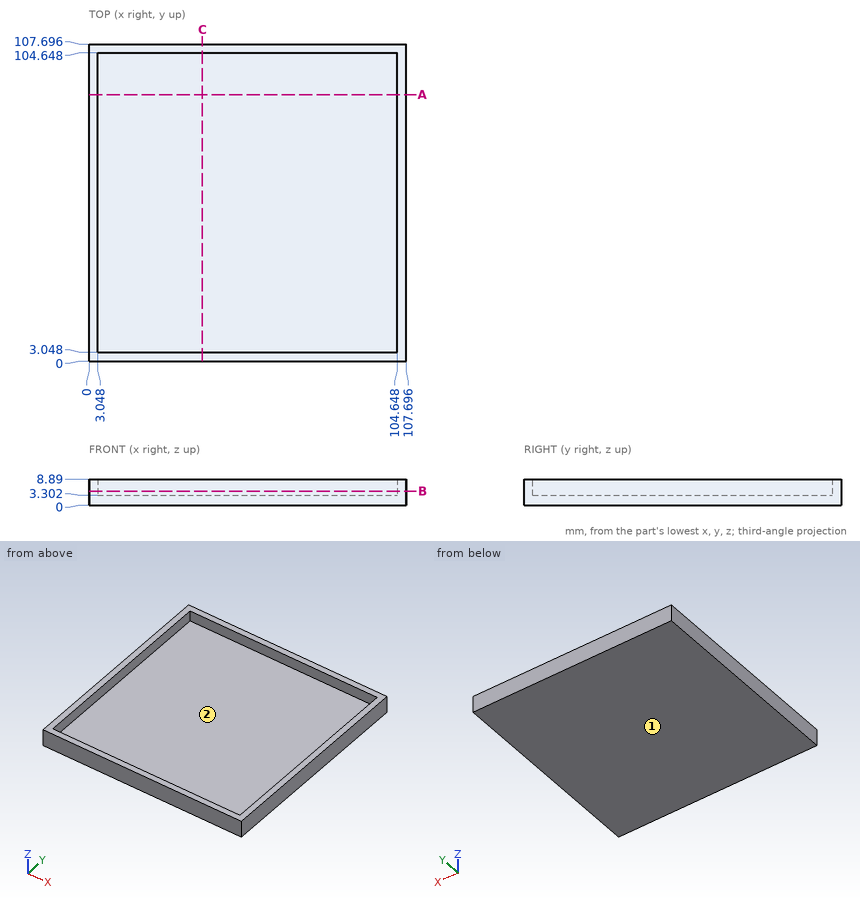
Job drawing, mm, ordinate dimensions from the low corner. One solid piece. Round coordinates to 2 decimals unless told otherwise and drop trailing zeros. Loops run counter-clockwise (first coordinate to the right, second up) from the corner with the lowest first, then second, coordinate; pieces in that order, holes last. Notation, with made-up numbers: (-1, 40) -> (23, 40) arc R22 cw to (23, 70) -> close; hole circle Ø10 at (77, 85.5). An arc over 180 degrees is marked (long way). One line per item, written item: value. Start each with the question number.
Q1. Probe line 1 along Y through (x, z) = (42.5, 4.25); line 2 along Z through (x, y) = (48, 60). List the from-to ranges inside material, lowest first.
Q2. Drop a flat-ended pin along its axis: pin 1 Ø1 at (x, y) = (95, 67) entering from +Z. Give the stop position or say it passes through.
Q3. Two-plate mould, pull along Y, no slides. Class the marked faces 1 and 2: released by +Y, released by -Y, zero draft, split by the parting line, or undercut.
Q4. Cut at B-B on z = 4.75. List the corners of the cut face in (x, y), plus the area to 3 significant figures.
Q5. Cut at A-A on y = 90.5. List the corners of the cut face in (x, z).
Computed:
1. line 1: 0 to 3.05, 104.65 to 107.7
1. line 2: 0 to 3.3
2. pin 1: z = 3.3
3. face 1: zero draft
3. face 2: undercut
4. outline: (0, 0) -> (107.7, 0) -> (107.7, 107.7) -> (0, 107.7) -> close; hole (3.05, 3.05) -> (104.65, 3.05) -> (104.65, 104.65) -> (3.05, 104.65) -> close
4. area: 1,280 mm²
5. outline: (0, 0) -> (107.7, 0) -> (107.7, 8.89) -> (104.65, 8.89) -> (104.65, 3.3) -> (3.05, 3.3) -> (3.05, 8.89) -> (0, 8.89) -> close
